Input: part model. Units: mm. Frame: model coordinates. A direction names the side the tool comes from. Round coordinates to 2 decimals unless told otherwise and drop trailing zeros. Order: outer loops, then holes, each group sorted by start corner. A loop starts at its lowest first (then second) coordinate and runs counter-clockwise, first axis right, second up. Notation, with made-up numbers: (-34, 43.5) -> (25, 43.5) arc R26 ccw to (25, 81.5) -> close; hole circle Ø10 at (71.25, 47.25). An arc over 180 degrees is marked (long way). Use a Markdown table: item, result.
Autodesk Inventor part; units mm, degrees
ref_plane "YZ Plane" through (0, 0, 0) normal (1, 0, 0) x (0, 1, 0)
ref_plane "XZ Plane" through (0, 0, 0) normal (0, 1, 0) x (-1, 0, 0)
ref_plane "XY Plane" through (0, 0, 0) normal (0, 0, 1) x (1, 0, 0)
sketch "Эскиз1" plane through (0, 0, 0) normal (0, 0, 1) x (1, 0, 0)
  line L0 (-4.7, 2.25) -> (4.7, 2.25)
  line L1 (4.7, 2.25) -> (4.7, -2.25)
  line L2 (4.7, -2.25) -> (-4.7, -2.25)
  line L3 (-4.7, -2.25) -> (-4.7, 2.25)
  point P0 (0, 0)
  point P1 (-4.7, 0)
  point P2 (0, 2.25)
  dimension "d0" = 9.4
  dimension "d1" = 4.5
extrude "Выдавливание1" add sketch "Эскиз1" along normal mid plane 10.2
sketch "Эскиз3" plane through (0, 0, 5.1) normal (0, 0, 1) x (1, 0, 0)
  line L0 (-4.7, 2.25) -> (-4.7, -2.25)
  line L1 (-4.7, 0.75) -> (-2.9, 0.75)
  line L2 (-2.9, 0.75) -> (-2.9, 2.25)
  line L3 (4.7, 2.25) -> (-4.7, 2.25)
  line L4 (4.7, -2.25) -> (4.7, 2.25)
  line L5 (4.7, 0.75) -> (2.9, 0.75)
  line L6 (2.9, 0.75) -> (2.9, 2.25)
  point P0 (0, 0)
  dimension "d7" = 1.5
  dimension "d8" = 2.9
  dimension "d9" = 5.8
extrude "Выдавливание2" cut sketch "Эскиз3" against normal blind 10.2
sketch "Эскиз5" plane through (0, 0, 5.1) normal (0, 0, 1) x (1, 0, 0)
  line L0 (-4.7, -2.25) -> (4.7, -2.25)
  line L1 (-2.9, -2.25) -> (-4.7, -0.75)
  line L2 (-4.7, 0.75) -> (-4.7, -2.25)
  line L3 (4.7, -2.25) -> (4.7, 0.75)
  line L4 (4.7, -0.75) -> (2.9, -2.25)
  point P0 (0, 0)
  dimension "d15" = 1.5
  dimension "d16" = 2.9
  dimension "d17" = 5.8
extrude "Выдавливание3" cut sketch "Эскиз5" against normal blind 10.2
sketch "Эскиз6" plane through (-2.9, 2.25, -5.1) normal (0, 1, 0) x (1, 0, 0)
  point P0 (2.9, -5.1)
  point P1 (2.9, -5.1)
hole "Отверстие1" at (0, 2.25, 0) direction (0, -1, 0) diameter 3 end through all
chamfer "Фаска1" distance 0.2 angle 45 2 edges at (0, 2.25, -1.5) (0, -2.25, -1.5)
fillet "Сопряжение2" radius 0.1 2 edges at (2.9, 2.25, 0) (-2.9, 2.25, 0)
fillet "Сопряжение3" radius 0.3 2 edges at (-4.7, 0.75, 0) (4.7, 0.75, 0)
thread "Резьба2"
properties part number "APM5N" material "Сталь"
1) Contact query for flat-ended pins moving along their axis: P1, Ø0.8, axis at x = 3.5, z = -2.5, coming from the +Y side; P2, Ø1.1, axis at y = 1.5, z = -2, coming from the +X side. Output: stop coordinate, or through.
Answer key:
| item | result |
|---|---|
| P1 | stops at y = 0.75 |
| P2 | stops at x = 2.9 |
2) Cut plane D-D on z = 3. Return loops of the section in (x, y), and give its area (3 significant figures).
Answer key:
| item | result |
|---|---|
| outline | (-4.7, -0.75) -> (-2.9, -2.25) -> (2.9, -2.25) -> (4.7, -0.75) -> (4.7, 0.45) arc R0.3 ccw to (4.4, 0.75) -> (2.9, 0.75) -> (2.9, 2.15) arc R0.1 ccw to (2.8, 2.25) -> (-2.8, 2.25) arc R0.1 ccw to (-2.9, 2.15) -> (-2.9, 0.75) -> (-4.4, 0.75) arc R0.3 ccw to (-4.7, 0.45) -> close |
| area | 34.2 mm^2 |
3) Draft query along Z for faces 1 (the face through (-3.8, -1.5, 0.1)), 2 (the face through (0, 0, 5.1)), 3 (the face through (-0.07, -0.03, -1.5)), 4 (the face through (0, 0, -5.1)). Return one class per face: released by +Z, released by -Z, zero draft, split by the parting line, or undercut.
Answer key:
| item | result |
|---|---|
| face 1 | zero draft |
| face 2 | released by +Z |
| face 3 | undercut |
| face 4 | released by -Z |
4) Set-up query: faces 5 (the face through (2.9, 1, 0)), 6 (the face through (-4.7, 0, 0)), 7 (the face through (-4, 0.75, 0)). Return all of +Z, -Z, +X, -X, +Y, -Y with unobstructed straight access to the full face (end or side cutting, diameter ignored); none if empty.
Answer key:
| item | result |
|---|---|
| face 5 | +Z, -Z, +X, +Y |
| face 6 | +Z, -Z, -X, +Y, -Y |
| face 7 | +Z, -Z, -X, +Y |
5) Cut plane B-B on z = 0. Return loops of the section in (x, y), and give its area (3 significant figures).
Answer key:
| item | result |
|---|---|
| outline | (-4.7, -0.75) -> (-2.9, -2.25) -> (-1.7, -2.25) -> (-1.5, -2.05) -> (-1.5, 2.05) -> (-1.7, 2.25) -> (-2.8, 2.25) arc R0.1 ccw to (-2.9, 2.15) -> (-2.9, 0.75) -> (-4.4, 0.75) arc R0.3 ccw to (-4.7, 0.45) -> close; (1.5, -2.05) -> (1.7, -2.25) -> (2.9, -2.25) -> (4.7, -0.75) -> (4.7, 0.45) arc R0.3 ccw to (4.4, 0.75) -> (2.9, 0.75) -> (2.9, 2.15) arc R0.1 ccw to (2.8, 2.25) -> (1.7, 2.25) -> (1.5, 2.05) -> close |
| area | 20.6 mm^2 |
6) Cut plane A-A on x = 0. Return loops of the section in (y, z), and give its area (3 significant figures).
Answer key:
| item | result |
|---|---|
| outline | (-2.25, -5.1) -> (2.25, -5.1) -> (2.25, -1.7) -> (2.05, -1.5) -> (-2.05, -1.5) -> (-2.25, -1.7) -> close; (-2.25, 1.7) -> (-2.05, 1.5) -> (2.05, 1.5) -> (2.25, 1.7) -> (2.25, 5.1) -> (-2.25, 5.1) -> close |
| area | 32.3 mm^2 |
7) Cut plane C-C on y = 1.75. Return loops of the section in (x, z), and give its area (3 significant figures).
Answer key:
| item | result |
|---|---|
| outline | (-2.9, -5.1) -> (2.9, -5.1) -> (2.9, 5.1) -> (-2.9, 5.1) -> close; hole circle Ø3 at (0, 0) |
| area | 52.1 mm^2 |
8) Ray query, probe 1 along X at (y, z) = (0.45, 0); probe 2 along Z at (x, y) = (0, 0.05); probe 3 along Z at (x, y) = (0.5, -0.1). Return the intervals inside material, ascending.
Answer key:
| item | result |
|---|---|
| probe 1 | x = -4.7 to -1.5, 1.5 to 4.7 |
| probe 2 | z = -5.1 to -1.5, 1.5 to 5.1 |
| probe 3 | z = -5.1 to -1.41, 1.41 to 5.1 |
